from build123d import *

# Parameters (mm, degrees)
SKETCH006_R     = 3.15
PAD002_DEPTH    = 190
SKETCH011_R     = 5
PAD007_DEPTH    = 50
SKETCH010_R     = 5
PAD006_DEPTH    = 50
SKETCH008_R     = 13
PAD004_DEPTH    = 15
SKETCH009_R     = 9
PAD005_DEPTH    = 15
SKETCH013_R     = 6
PAD008_DEPTH    = 26
BOX001_W        = 50
BOX001_H        = 180
BOX001_DEPTH    = 20
SKETCH015_R     = 1.5
POCKET001_DEPTH = 395.766885
SKETCH016_R     = 1.5
POCKET002_DEPTH = 395.766885
SKETCH017_R     = 3
POCKET003_DEPTH = 5
SKETCH018_R     = 3
POCKET004_DEPTH = 5


with BuildPart() as pad002:
    # Sketch006 → Pad002 (new body)
    with BuildSketch(Plane.XZ.offset(80)):
        Circle(SKETCH006_R)
    extrude(amount=-PAD002_DEPTH)


with BuildPart() as pad007:
    # Sketch011 → Pad007 (new body)
    with BuildSketch(Plane.XZ.offset(-75)):
        Circle(SKETCH011_R)
    extrude(amount=PAD007_DEPTH)


with BuildPart() as scassi_perno:
    # Sketch010 → Pad006 (new body)
    with BuildSketch(Plane.XZ.offset(25)):
        Circle(SKETCH010_R)
    extrude(amount=PAD006_DEPTH)

    # Fusion002: union Pad007
    add(pad007.part)


with BuildPart() as scasso_ruota_dentata:
    # Sketch008 → Pad004 (new body)
    with BuildSketch(Plane.XZ.offset(-3)):
        Circle(SKETCH008_R)
    extrude(amount=PAD004_DEPTH)


with BuildPart() as obj1:
    # Sketch009 → Pad005 (new body)
    with BuildSketch(Plane.XZ.offset(-3)):
        with Locations((15.997087, 9e-06)):
            Circle(SKETCH009_R)
    extrude(amount=PAD005_DEPTH)

    # Fusion001: union scasso_ruota_dentata
    add(scasso_ruota_dentata.part)


with BuildPart() as fusion:
    # Sketch013 → Pad008 (new body)
    with BuildSketch(Plane.XZ.offset(11)):
        with Locations((16.059561, 9e-06)):
            Circle(SKETCH013_R)
    extrude(amount=PAD008_DEPTH)

    # Fusion005: union scassi_perno, obj1
    add(scassi_perno.part)
    add(obj1.part)

    # Fusion: union Pad002
    add(pad002.part)


with BuildPart() as obj2:
    # Box001 → Box001 (new body)
    with BuildSketch(Plane(origin=(-20, -88, -21), x_dir=(1, 0, 0), z_dir=(0, 0, 1))):
        with Locations((25, 90)):
            Rectangle(BOX001_W, BOX001_H)
    extrude(amount=BOX001_DEPTH)

    # Cut001: cut Fusion
    add(fusion.part, mode=Mode.SUBTRACT)

    # Sketch015 → Pocket001 (cut, through all)
    with BuildSketch(Plane(origin=(0, 0, -21), x_dir=(1, 0, 0), z_dir=(0, 0, -1))):
        with Locations((23, 70)):
            Circle(SKETCH015_R)
    pocket001 = extrude(amount=-POCKET001_DEPTH, mode=Mode.SUBTRACT)

    # Mirrored: Pocket001 across Sketch015 H_Axis
    add(pocket001.mirror(Plane(origin=(0, 0, -21), x_dir=(0, 0, -1), z_dir=(0, -1, 0))), mode=Mode.SUBTRACT)

    # Sketch016 → Pocket002 (cut, through all)
    with BuildSketch(Plane(origin=(0, 0, -21), x_dir=(1, 0, 0), z_dir=(0, 0, -1))):
        with Locations((-12, 70)):
            Circle(SKETCH016_R)
    pocket002 = extrude(amount=-POCKET002_DEPTH, mode=Mode.SUBTRACT)

    # Mirrored001: Pocket002 across Sketch016 H_Axis
    add(pocket002.mirror(Plane(origin=(0, 0, -21), x_dir=(0, 0, -1), z_dir=(0, -1, 0))), mode=Mode.SUBTRACT)

    # Sketch017 → Pocket003 (cut)
    with BuildSketch(Plane(origin=(0, 0, -21), x_dir=(1, 0, 0), z_dir=(0, 0, -1))):
        with Locations((23, 70)):
            Circle(SKETCH017_R)
    pocket003 = extrude(amount=-POCKET003_DEPTH, mode=Mode.SUBTRACT)

    # Mirrored002: Pocket003 across Sketch017 H_Axis
    add(pocket003.mirror(Plane(origin=(0, 0, -21), x_dir=(0, 0, -1), z_dir=(0, -1, 0))), mode=Mode.SUBTRACT)

    # Sketch018 → Pocket004 (cut)
    with BuildSketch(Plane(origin=(0, 0, -21), x_dir=(1, 0, 0), z_dir=(0, 0, -1))):
        with Locations((-12, 70)):
            Circle(SKETCH018_R)
    pocket004 = extrude(amount=-POCKET004_DEPTH, mode=Mode.SUBTRACT)

    # Mirrored003: Pocket004 across Sketch018 H_Axis
    add(pocket004.mirror(Plane(origin=(0, 0, -21), x_dir=(0, 0, -1), z_dir=(0, -1, 0))), mode=Mode.SUBTRACT)


solid = obj2.part
Build history of the part. All positions in model axes, mm. A direction names the side the tool comes from. Coordinates: 2 decimals unless noted, no trailing zeros. Order: outer loops, then holes, each group sorted by start corner. A loop starts at its lowest first (then second) coordinate and runs counter-clockwise, first axis right, second up. Notation, with made-up numbers: M -35,40.5 L 21,40.5 A16 ccw 21,65.5 Z; hole C 65.5,-13 d11. An arc over 180 degrees is marked long. One line per question, with ' | ' between items. Start each with the question number.
Q1. Saw through at C-C (y = 46). List the corners of the cut face in (x, z).
Q2. Two-plate mould, pull along Y, no slides. Class faces 1 (the face through (0, 50, -5)), 2 (the face through (5, -88, -11)), 3 (the face through (-0.06, 13.85, -3.15)): +Y half, -Y half, draft (parallel to the pull), parting line (faces both ways), or undercut.
Q3. Flat gauge pins, fed straight in: pin 1 Ø3.5 at (x, y) = (23, 70) entering from -Z; pin 2 Ø1.8 at (x, y) = (-12, 70) entering from -Z. Where does each tip first touch, or does it go through?
Q4. Probe L1, parallel to X at y = -70, z = -6; L2, parallel to X at y = -70, z = -18.55; L3, parallel to Y at x = 23, z = -7.75. List the from-to ranges inside material, lowest first. Write a range as from..to.
Q5. Saw through at B-B (x = 17). List the corners of the cut face in (y, z), then the cut area to 3 significant figures.
Q6. Saw through at D-D (x = -7). List the corners of the cut face in (y, z), then the cut area to 3 significant figures.
Q7. 3-axis set-ups, long thin cutter, end or side, ignore diameter. For faces 4 (the face through (22.35, -67.07, -18.54)), 5 (the face through (-0.06, -77.54, -3.15)), 6 (the face through (-0.1, -25, -3.4)): which of +Z, -Z, +X, -X, +Y, -Y reach the whole face in a straight line?
Q8. Saw through at A-A (y = -17). List the corners of the cut face in (x, z), then the cut area to 3 significant figures.
Check values:
1) outline: M -20,-21 L 30,-21 L 30,-1 L 4.9,-1 A5 cw -4.9,-1 L -20,-1 Z
2) face 1: undercut | face 2: -Y half | face 3: draft
3) pin 1: stops at z = -16 | pin 2: passes through
4) L1: x = -20..-13.5, -10.5..21.5, 24.5..30 | L2: x = -20..-15, -9..20, 26..30 | L3: y = -88..-71.5, -68.5..68.5, 71.5..92
5) outline: M -88,-21 L 92,-21 L 92,-1 L 3,-1 L 3,-8.94 L -12,-8.94 L -12,-5.93 L -37,-5.93 L -37,-1 L -88,-1 Z | area: 3,360 mm2
6) outline: M -88,-21 L 92,-21 L 92,-1 L 3,-1 L 3,-10.95 L -12,-10.95 L -12,-1 L -88,-1 Z | area: 3,450 mm2
7) face 4: -Z | face 5: +Z, +Y | face 6: +Z
8) outline: M -20,-21 L 30,-21 L 30,-1 L 21.98,-1 A6 cw 10.14,-1 L 2.99,-1 A3.15 cw -2.99,-1 L -20,-1 Z | area: 946 mm2
